Geometry check sheet. Reference: drawing and pictorial views, mm from the part's lowest x, y, z. A direction names the side the tool comes from. Round coordinates to 2 decimals unless told otherwise and drop trailing zeros. Order: outer loops, then holes, each group sorted by start corner. A loop starts at its lowest first (then second) coordinate and runs counter-clockwise, first axis right, second up. Notation, with made-up numbers: (38, 60.5) -> (56, 60.5) arc R29 cw to (56, 85.5) -> close; hole circle Ø7 at (84, 86). An arc over 180 degrees is marked (long way). Put each result on its own line as item: value.
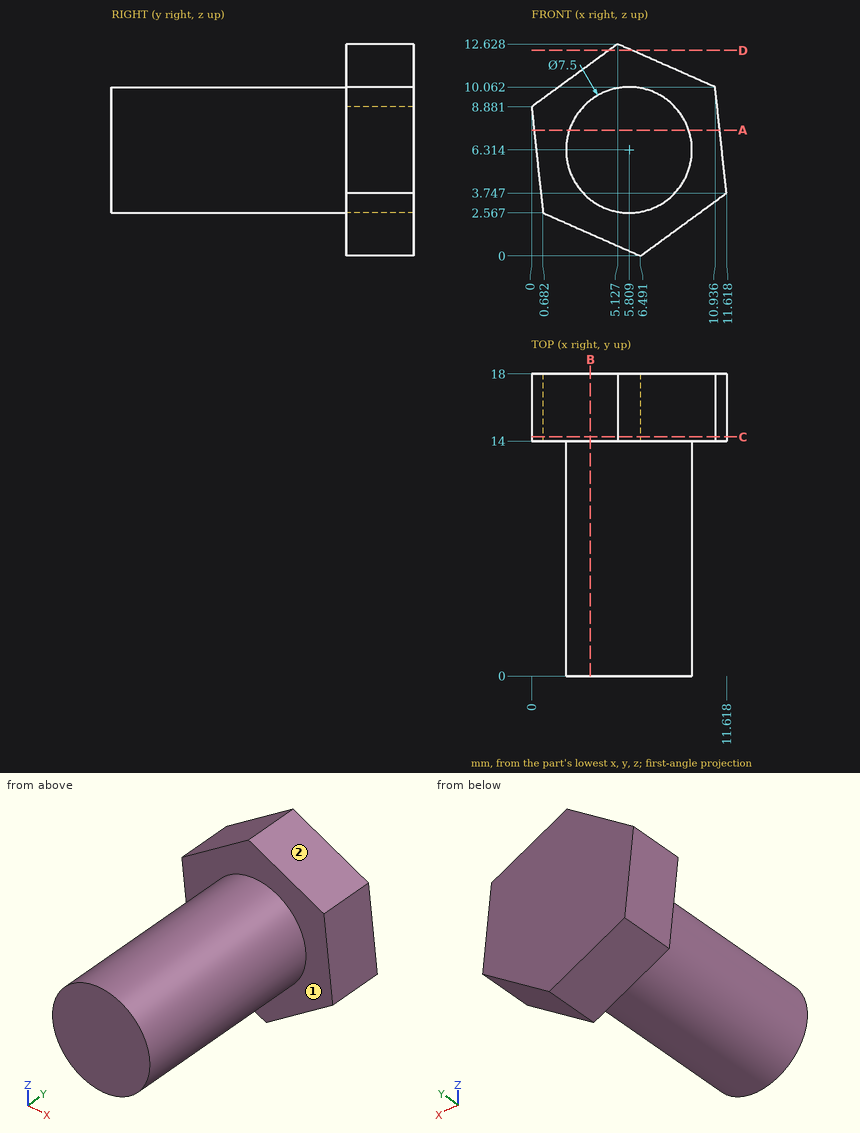
Item 1: Sectioned sample at C-C, the plane y = 14.25. Record the boundary of the cut face in (x, z).
Geometry check:
outline: (0, 8.88) -> (0.68, 2.57) -> (6.49, 0) -> (11.62, 3.75) -> (10.94, 10.06) -> (5.13, 12.63) -> close
Item 2: Depth check by flat-ended pin: pin 1 Ø4 at (x, y) = (8, 9) entering from +Z; pin 2 Ø2 at (y, z) = (3, 9.5) entering from +X (1 decimal); pin 3 Ø3 at (x, y) = (10.5, 14.5) entering from +Z. Enter the tip coordinate at first touch or a pass-through.
Geometry check:
pin 1: z = 10.06
pin 2: x = 8.9
pin 3: z = 10.92
Item 3: Sectioned sample at B-B, the plane x = 3.5. Record the boundary of the cut face in (y, z), then the cut area to 3 significant figures.
Geometry check:
outline: (0, 3.36) -> (14, 3.36) -> (14, 1.32) -> (18, 1.32) -> (18, 11.44) -> (14, 11.44) -> (14, 9.27) -> (0, 9.27) -> close
area: 123 mm2
Item 4: Tool access check on the marked faces 1 and 2. Record the directions out of +Z, -Z, +X, -X, +Y, -Y that give a thin tool (end or side, any length) a straight path to the whole face; none if there is none.
Geometry check:
face 1: -Y
face 2: +Z, +X, +Y, -Y
Item 5: Material ranges on line 1 along Y through (x, z) = (7, 10.5); line 2 along X through (y, z) = (17.75, 2.5) (1 decimal); line 3 along Z through (x, y) = (6.25, 11.75), recorded low to high.
Geometry check:
line 1: 14 to 18
line 2: 0.8 to 9.9
line 3: 2.59 to 10.04
Item 6: Sectioned sample at D-D, the plane z = 12.25. Record the boundary of the cut face in (x, y).
Geometry check:
outline: (4.61, 14) -> (5.98, 14) -> (5.98, 18) -> (4.61, 18) -> close
Item 7: Sectioned sample at A-A, the plane z = 7.5. Record the boundary of the cut face in (x, y), then the cut area to 3 significant figures.
Geometry check:
outline: (0.15, 14) -> (2.25, 14) -> (2.25, 0) -> (9.37, 0) -> (9.37, 14) -> (11.21, 14) -> (11.21, 18) -> (0.15, 18) -> close
area: 144 mm2
